from build123d import *

# Parameters (mm, degrees)
F0_R     = 26.9875
F1_DEPTH = 9.525
F2_DEPTH = 4.7625
F3_R     = 12.7
F4_R     = 6.35
F5_DEPTH = 9.526
F6_R     = 5.08


with BuildPart() as f1:
    # F0 (on Front) → F1 (new body)
    with BuildSketch(Plane.XZ):
        Polygon((0, 76.2), (0, 0), (266.7, 0), (266.7, 22.225), (368.3, 22.225), (368.3, 53.975), (266.7, 53.975), (266.7, 76.2), align=None)
        with Locations((34.925, 38.1)):
            Circle(F0_R, mode=Mode.SUBTRACT)
        with Locations((98.425, 38.1)):
            Circle(F0_R, mode=Mode.SUBTRACT)
        with Locations((161.925, 38.1)):
            Circle(F0_R, mode=Mode.SUBTRACT)
        with Locations((225.425, 38.1)):
            Circle(F0_R, mode=Mode.SUBTRACT)
        with Locations((34.925, 38.1)):
            Circle(F0_R)
        with Locations((98.425, 38.1)):
            Circle(F0_R)
        with Locations((161.925, 38.1)):
            Circle(F0_R)
        with Locations((225.425, 38.1)):
            Circle(F0_R)
    extrude(amount=F1_DEPTH)

    # F0 (on Front) → F2 (cut)
    with BuildSketch(Plane.XZ):
        with Locations((225.425, 38.1)):
            Circle(F0_R)
        with Locations((161.925, 38.1)):
            Circle(F0_R)
        with Locations((98.425, 38.1)):
            Circle(F0_R)
        with Locations((34.925, 38.1)):
            Circle(F0_R)
    extrude(amount=F2_DEPTH, mode=Mode.SUBTRACT)

    # F3
    f3_edges = [f1.edges().sort_by_distance(p)[0] for p in [
        (0, -4.7625, 76.2),
        (0, -4.7625, 0),
        (266.7, -4.7625, 76.2),
        (266.7, -4.7625, 0),
        (368.3, -4.7625, 53.975),
        (368.3, -4.7625, 22.225),
    ]]
    fillet(f3_edges, radius=F3_R)

    # F4 (on face) → F5 (cut, through all)
    with BuildSketch(Plane(origin=(0, 0, 0), x_dir=(-1, 0, 0), z_dir=(0, 1, 0))):
        with Locations((-349.25, 38.1)):
            Circle(F4_R)
    extrude(amount=-F5_DEPTH, mode=Mode.SUBTRACT)

    # F6
    f6_edges = [f1.edges().sort_by_distance(p)[0] for p in [
        (266.7, -4.7625, 53.975),
        (266.7, -4.7625, 22.225),
    ]]
    fillet(f6_edges, radius=F6_R)


solid = f1.part
Here's how the part is built. I have some questions about the finished solid (model axes, mm). A direction names the side the tool comes from. Give positions to 0.01 mm unless a question says otherwise; leave off trailing zeros. Loops run counter-clockwise (first coordinate to the right, second up) from the corner with the lowest first, then second, coordinate; pieces in that order, holes last. Notation, with made-up numbers: (-18, 23) -> (39, 23) arc R22 cw to (39, 40) -> close; hole circle Ø3 at (-31, 52.25). An arc over 180 degrees is marked (long way). Answer as a JSON object with one key per item and string values. Group by question number.
Item 1: I need wall thicknesses on L1, parallel to Z at x = 160, y = -0.25; L2, parallel to X at y = -2.5, z = 16; L3, parallel to X at y = -0.75, z = 43.5. Which ranges of each line are inside material? Lowest first, please.
Item 2: Imagine slicing it at B-B on x = 349.25. Write out the boundary of the cut face in (y, z) (3 decimals).
Item 3: Imagine slicing it at A-A on z = 38.1. Write out the boundary of the cut face in (x, y) (1 decimal).
Item 4: Imagine slicing it at C-C on y = -7. Write out the boundary of the cut face in (x, z) (3 decimals).
Item 5: On a 3-axis mill with a long thin cutter (end or side, diameter ignored), from which of +Z, -Z, +X, -X, +Y, -Y can I reach the whole of each face in a straight line? I mean faces 4 (the cylindrical face through (250.355, -2.348, 27.764)), 5 (the cylindrical face through (262.88, -4.83, 72.58)), 6 (the flat face through (313, -5, 22.225)). Say none if no direction works.
Item 6: Imagine slicing it at D-D on x = 239. Write out the boundary of the cut face in (y, z) (1 decimal), then the cut area to 3 significant figures.
Item 7: Will these pins go through, and if not, where does the flat tip stop? pin 1 (16 mm diameter, centred on x = 92, z = 29.5, fed in from +Y); pin 2 (3 mm diameter, centred on x = 325.5, y = -5, fed in from -Z) (3 decimals); pin 3 (4 mm diameter, centred on y = -6, z = 11.5, fed in from +X).
Item 8: Thinking about a two-plate mould opening in X: for faces 1 (the cylindrical face through (355.594, -4.696, 38.379)), 2 (the flat face through (314, -5, 53.975)), 3 (the cylindrical face through (3.62, -4.83, 72.38)), which applies, pulls with the +X half, pulls with the -X half, needs draft (parallel to the pull), parting line crosses it, or undercut?
Answer list:
{
 "1": {"L1": "z = 0 to 11.18, 65.02 to 76.2", "L2": "x = 0 to 19.44, 50.41 to 82.94, 113.91 to 146.44, 177.41 to 209.94, 240.91 to 266.7", "L3": "x = 0 to 8.48, 61.37 to 71.98, 124.87 to 135.48, 188.37 to 198.98, 251.87 to 345.91, 352.59 to 368.1"},
 "2": {"outline": "(-9.525, 22.225) -> (0, 22.225) -> (0, 31.75) -> (-9.525, 31.75) -> close; (-9.525, 44.45) -> (0, 44.45) -> (0, 53.975) -> (-9.525, 53.975) -> close"},
 "3": {"outline": "(0, -9.5) -> (342.9, -9.5) -> (342.9, 0) -> (252.4, 0) -> (252.4, -4.8) -> (198.4, -4.8) -> (198.4, 0) -> (188.9, 0) -> (188.9, -4.8) -> (134.9, -4.8) -> (134.9, 0) -> (125.4, 0) -> (125.4, -4.8) -> (71.4, -4.8) -> (71.4, 0) -> (61.9, 0) -> (61.9, -4.8) -> (7.9, -4.8) -> (7.9, 0) -> (0, 0) -> close; (355.6, -9.5) -> (368.3, -9.5) -> (368.3, 0) -> (355.6, 0) -> close"},
 "4": {"outline": "(0, 12.7) arc R12.7 ccw to (12.7, 0) -> (254, 0) arc R12.7 ccw to (266.7, 12.7) -> (266.7, 17.145) arc R5.08 cw to (271.78, 22.225) -> (355.6, 22.225) arc R12.7 ccw to (368.3, 34.925) -> (368.3, 41.275) arc R12.7 ccw to (355.6, 53.975) -> (271.78, 53.975) arc R5.08 cw to (266.7, 59.055) -> (266.7, 63.5) arc R12.7 ccw to (254, 76.2) -> (12.7, 76.2) arc R12.7 ccw to (0, 63.5) -> close; hole circle Ø12.7 at (349.25, 38.1)"},
 "5": {"face 4": "+Y", "face 5": "+Z, +X, +Y, -Y", "face 6": "-Z, +X, +Y, -Y"},
 "6": {"outline": "(-9.5, 0) -> (0, 0) -> (0, 14.8) -> (-4.8, 14.8) -> (-4.8, 61.4) -> (0, 61.4) -> (0, 76.2) -> (-9.5, 76.2) -> close", "area": "504 mm2"},
 "7": {"pin 1": "stops at y = -4.76", "pin 2": "stops at z = 22.225", "pin 3": "stops at x = 266.7"},
 "8": {"face 1": "undercut", "face 2": "needs draft", "face 3": "pulls with the -X half"}
}
